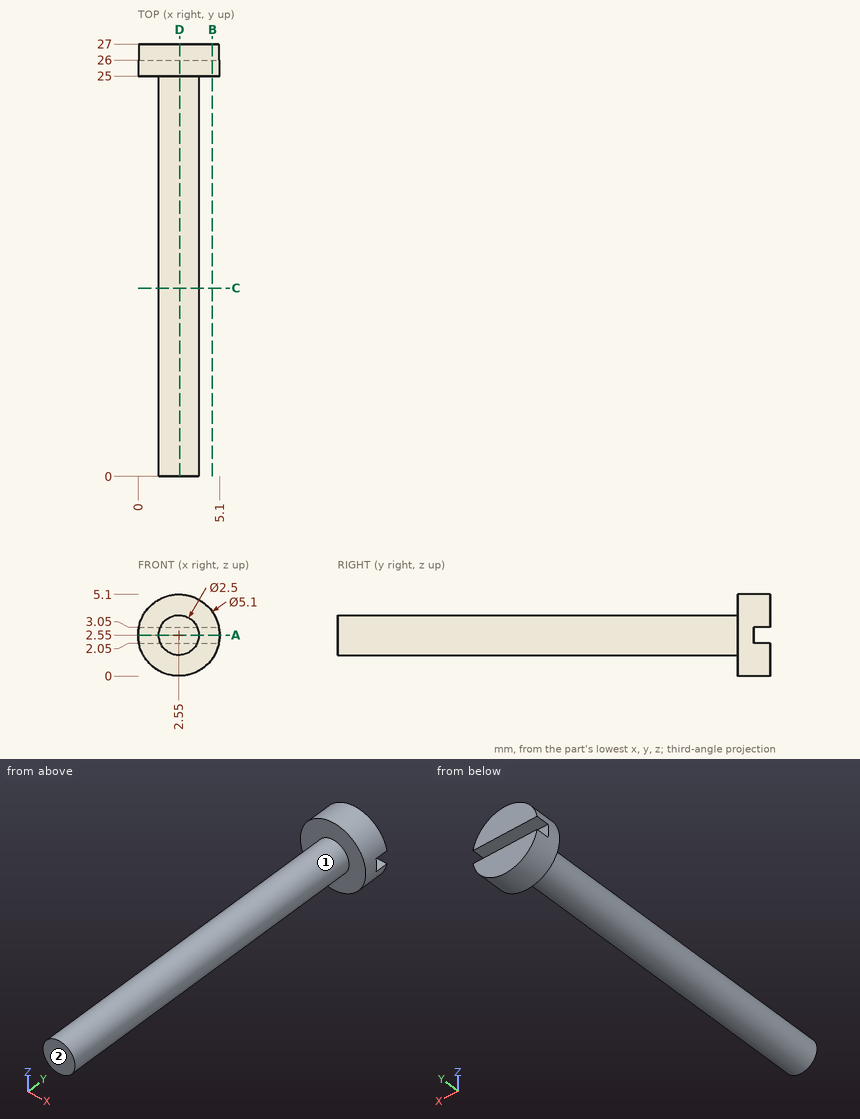
Study the drawing (mm; zero at the part's minimum x, y, z) and answer. A direction names the side the tool comes from. Round coordinates to 2 decimals unless told otherwise and drop trailing zeros. Loops run counter-clockwise (first coordinate to the right, second up) from the corner with the lowest first, then second, coordinate; pieces in that order, holes last. Notation, with made-up numbers: M 10,64.25 L 63,64.25 A18 cw 63,77.25 Z; hole C 56,89.25 d2. An arc over 180 degrees is marked long. One line per question, with ' | ' between items.
Q1. Find section B-B, the plane x = 4.65. Give the vertices of the cut face in (y, z), then the cut area to 3 significant figures.
Conclusion:
outline: M 25,1.1 L 27,1.1 L 27,2.05 L 26,2.05 L 26,3.05 L 27,3.05 L 27,4 L 25,4 Z | area: 4.79 mm2
Q2. Find section D-D, the plane x = 2.6. Give the vertices of the cut face in (y, z).
Conclusion:
outline: M 0,1.3 L 25,1.3 L 25,0 L 27,0 L 27,2.05 L 26,2.05 L 26,3.05 L 27,3.05 L 27,5.1 L 25,5.1 L 25,3.8 L 0,3.8 Z
Q3. A tool of negligible diameter and unlimited length cuts with its end or side. For the marked faces 1 and 2, from which of +Z, -Z, +X, -X, +Y, -Y can it reach the whole face along a straight path? Write none if from no direction.
Conclusion:
face 1: -Y | face 2: +Z, -Z, +X, -X, -Y
Q4. Find section A-A, the plane z = 2.55. Give the vertices of the cut face in (x, y), then the cut area to 3 significant figures.
Conclusion:
outline: M 0,25 L 1.3,25 L 1.3,0 L 3.8,0 L 3.8,25 L 5.1,25 L 5.1,26 L 0,26 Z | area: 67.6 mm2
Q5. Consider line 1 along Y through (x, z) = (2.85, 4.9); line 2 along X through (y, z) = (6.75, 2.6); line 3 along Y through (x, z) = (0.35, 2.3). Determine where each line is inside the solid, lowest interval first. Write a range as from..to.
Conclusion:
line 1: y = 25..27 | line 2: x = 1.3..3.8 | line 3: y = 25..26
Q6. Find section C-C, the plane y = 11.75. Give the vertices of the cut face in (x, z).
Conclusion:
outline: C 2.55,2.55 d2.5
Q7. Each of these flat-tipped pins is pushed along its axis until it touches: pin 1 Ø0.8 at (x, y) = (2, 26.5) entering from -Z; pin 2 Ø1.5 at (y, z) = (12.5, 3.5) entering from +X; pin 3 Ø1.5 at (y, z) = (20.5, 3) entering from -X. Where does it stop, or does it pass through?
Conclusion:
pin 1: stops at z = 0 | pin 2: stops at x = 3.78 | pin 3: stops at x = 1.3
